from build123d import *

# Parameters (mm, degrees)
F0_W     = 80
F0_H     = 100
F1_DEPTH = 150
F2_R     = 20
F3_DEPTH = 141.9
F4_R     = 8
F5_W     = 134
F5_H     = 84
F6_DEPTH = 1.6


with BuildPart() as f1:
    # F0 (on Front) → F1 (new body)
    with BuildSketch(Plane.XZ):
        Rectangle(F0_W, F0_H)
    extrude(amount=F1_DEPTH)

    # F2 (on face) → F3 (cut, symmetric)
    with BuildSketch(Plane.XY.offset(50)):
        with Locations((0, -72.1363547525)):
            Circle(F2_R)
    extrude(amount=F3_DEPTH, both=True, mode=Mode.SUBTRACT)

    # F4
    f4_edges = [f1.edges().sort_by_distance(p)[0] for p in [
        (40, -75, 50),
        (0, 0, 50),
        (0, -150, 50),
        (-40, -75, 50),
        (-20, -72.136355, 50),
        (0, -150, -50),
        (40, -150, 0),
        (-40, -150, 0),
        (40, -75, -50),
        (40, 0, 0),
        (-40, -75, -50),
        (0, 0, -50),
        (-20, -72.136355, -50),
        (-40, 0, 0),
    ]]
    fillet(f4_edges, radius=F4_R)

    # F5 (on face) → F6 (cut)
    with BuildSketch(Plane.YZ.offset(40)):
        with Locations((-75, 0)):
            Rectangle(F5_W, F5_H)
        with BuildLine():
            Line((-116.0339047565, -5.6421386253), (-126.7773912041, -5.6421386253))
            Line((-126.7773912041, -5.6421386253), (-126.7773912041, -27.0390193909))
            Line((-126.7773912041, -27.0390193909), (-132.7572563023, -27.0390193909))
            Line((-132.7572563023, -27.0390193909), (-132.7572563023, 24.4148480924))
            Line((-132.7572563023, 24.4148480924), (-118.6465765131, 24.4148480924))
            add(Edge.make_bspline(
                [(-118.6465765131, 24.4148480924), (-109.1756413953, 24.4148480924), (-104.654142644, 20.7886398784)],
                knots=[0, 0, 0, 1, 1, 1], degree=2))
            add(Edge.make_bspline(
                [(-104.654142644, 20.7886398784), (-100.1326438927, 17.1624316645), (-100.1326438927, 9.876230688)],
                knots=[0, 0, 0, 1, 1, 1], degree=2))
            add(Edge.make_bspline(
                [(-100.1326438927, 9.876230688), (-100.1326438927, -0.3267029824), (-110.4819772736, -3.9191266478)],
                knots=[0, 0, 0, 1, 1, 1], degree=2))
            Line((-110.4819772736, -3.9191266478), (-96.5064356787, -27.0390193909))
            Line((-96.5064356787, -27.0390193909), (-103.5786678476, -27.0390193909))
            Line((-103.5786678476, -27.0390193909), (-116.0339047565, -5.6421386253))
        make_face(mode=Mode.SUBTRACT)
        Polygon((-59.5236165027, -21.6897991995), (-59.5236165027, -27.0390193909), (-88.2066982449, -27.0390193909), (-88.2066982449, 24.4148480924), (-59.5236165027, 24.4148480924), (-59.5236165027, 19.0994124496), (-82.2268331467, 19.0994124496), (-82.2268331467, 2.5224606143), (-60.8975214782, 2.5224606143), (-60.8975214782, -2.75919048), (-82.2268331467, -2.75919048), (-82.2268331467, -21.6897991995), align=None, mode=Mode.SUBTRACT)
        Polygon((-48.656253377, 24.4148480924), (-35.0298187841, -1.3177164074), (-21.3132920617, 24.4148480924), (-14.837920251, 24.4148480924), (-32.0117324445, -7.0836126979), (-32.0117324445, -27.0390193909), (-38.0591666399, -27.0390193909), (-38.0591666399, -7.3651506027), (-55.1991942848, 24.4148480924), align=None, mode=Mode.SUBTRACT)
    extrude(amount=-F6_DEPTH, mode=Mode.SUBTRACT)


solid = f1.part
Can you work these out from the model? Positions are in its coordinate system, mm. A direction names the side the tool comes from. Give positions to 0.01 mm unless a question says otherwise; leave off trailing zeros. Loops run counter-clockwise (first coordinate to the right, second up) from the corner with the lowest first, then second, coordinate; pieces in that order, holes last. Notation, with made-up numbers: (17.25, 74.25) - (67.25, 74.25) arc R21 ccw to (67.25, 99.25) - close; hole circle Ø1 at (-37, 20.25). An arc over 180 degrees is marked (long way). Answer as a JSON object with one key per item and string values.
Q1. Will these pins go through, and if not, where does the flat tip stop? P1, Ø1.3, axis at x = 39, y = -129, coming from the -Z side; P2, Ø0.8, axis at x = 39, y = -18.5, coming from the +Z side; P3, Ø1.3, axis at x = 39.5, y = -122.5, coming from the -Z side.
Geometry says:
{"P1": "z = -46.87", "P2": "z = 46.52", "P3": "z = -46.13"}
Q2. If I drill on L1, parallel to Y at x = 0, z = 25; L2, parallel to X at y = -71, z = -25.5; L3, parallel to X at y = -110, z = 41, over which ranges is the centre line in solid material (lowest first)?
Geometry says:
{"L1": "-150 to -92.14, -52.14 to 0", "L2": "-40 to -19.97, 19.97 to 40", "L3": "-40 to 38.4"}
Q3. Imagine slicing it at B-B on z = 27.5. Write out the boundary of the cut face in (x, y).
Geometry says:
{"outline": "(-40, -142) arc R8 ccw to (-32, -150) - (32, -150) arc R8 ccw to (40, -142) - (38.4, -142) - (38.4, -8) - (40, -8) arc R8 ccw to (32, 0) - (-32, 0) arc R8 ccw to (-40, -8) - close; hole circle Ø40 at (0, -72.14)"}
Q4. Which directions (+Z, -Z, +X, -X, +Y, -Y) give clear straight access to the entire face, cutting with the end or side of a thin tool? Please do faces 4 (the flat face through (39.21, -109.72, -16.49)), 5 (the cylindrical face through (0.448, -2.406, 47.719)).
Geometry says:
{"face 4": "+X", "face 5": "+Z, +X, -X, +Y"}
Q5. If we mould it in two halves opening along Y, with no side actions, what happens to faces 1 (the flat face through (39.21, -41.94, 11.73)), 2 (the cylindrical face through (-37.719, -2.406, 0.588)), 3 (the cylindrical face through (-37.719, -75.938, 47.594))? For each: pulls with the +Y half, pulls with the -Y half, needs draft (parallel to the pull), parting line crosses it, or undercut.
Geometry says:
{"face 1": "undercut", "face 2": "pulls with the +Y half", "face 3": "needs draft"}
Q6. Imagine slicing it at A-A on x = 0. Write out the boundary of the cut face in (y, z).
Geometry says:
{"outline": "(-150, -42) arc R8 ccw to (-142, -50) - (-100.14, -50) arc R8 ccw to (-92.14, -42) - (-92.14, 42) arc R8 ccw to (-100.14, 50) - (-142, 50) arc R8 ccw to (-150, 42) - close; (-52.14, -42) arc R8 ccw to (-44.14, -50) - (-8, -50) arc R8 ccw to (0, -42) - (0, 42) arc R8 ccw to (-8, 50) - (-44.14, 50) arc R8 ccw to (-52.14, 42) - close"}
